Part print with two shaded views. Sizes in mm from the minimum x, y, z corner. A direction names the side the tool comes from. Coordinates: 2 decimals unless noted, no trailing zeros. Order: outer loops, then holes, each group sorted by start corner. A loop starts at its lowest first (then second) coordinate and runs counter-clockwise, first axis right, second up.
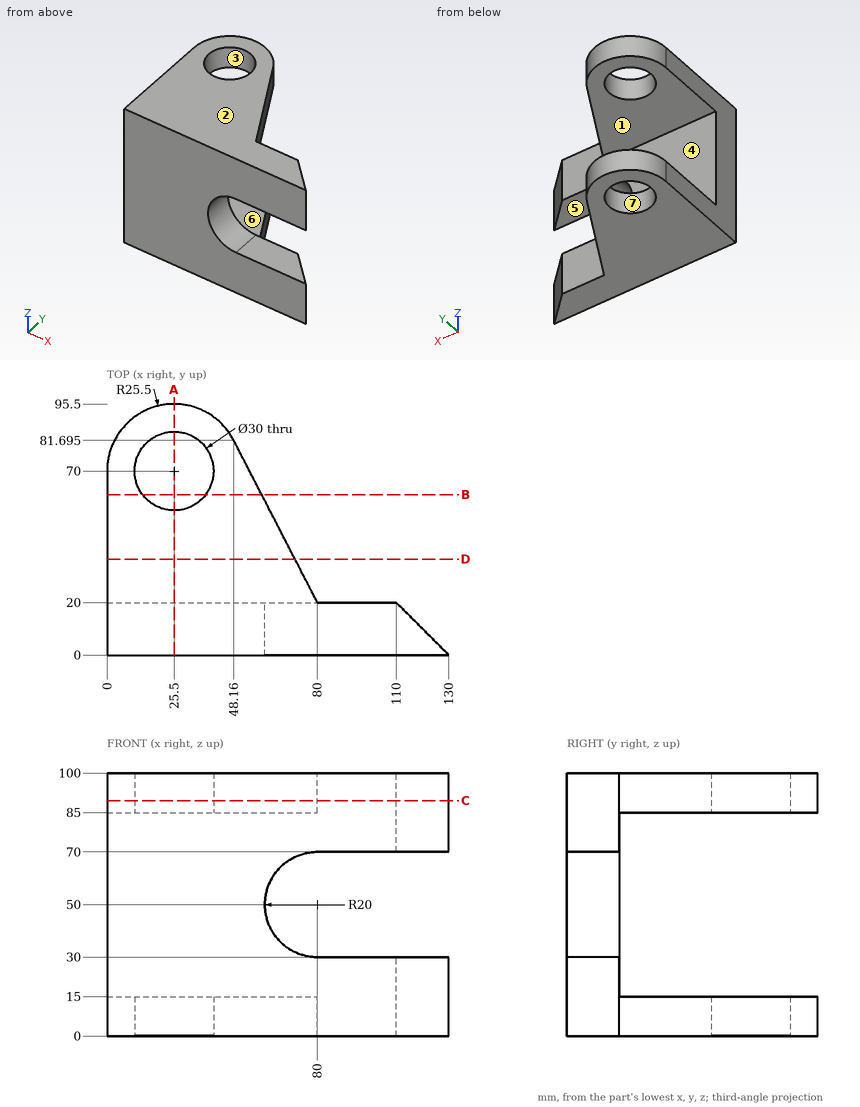
Q1. Wall check: line 1 along Y through (x, z) = (25.5, 9.75); line 2 along Z through (x, y) = (58, 46.5); line 3 along Y through (x, z) = (108, 13). Give the ranges that are in metal, low to high.
Results list:
line 1: y = 0 to 55, 85 to 95.5
line 2: z = 0 to 15, 85 to 100
line 3: y = 0 to 20
Q2. Cut at D-D on y = 36.5. Write the cut outline in (x, z) (1 decimal), and give its area (3 significant figures).
Results list:
outline: (0, 0) - (71.5, 0) - (71.5, 15) - (0, 15) - close; (0, 85) - (71.5, 85) - (71.5, 100) - (0, 100) - close
area: 2,140 mm2
Q3. Pin check, flat tips, straight feed: pin 1 Ø24 at (x, y) = (25.5, 70) entering from +Z; pin 2 Ø8 at (x, z) = (83, 12.5) entering from +Y. Stop position of each tip, or through.
Results list:
pin 1: passes through
pin 2: stops at y = 21.94
Q4. Mould opens along Z. For the marked faces 1, 2, 3 and 4 say: pulls with the +Z half, pulls with the -Z half, needs draft (parallel to the pull), parting line crosses it, or undercut.
Results list:
face 1: undercut
face 2: pulls with the +Z half
face 3: needs draft
face 4: undercut
Q5. Cut at A-A on x = 25.5. Write the cut outline in (y, z).
Results list:
outline: (0, 0) - (55, 0) - (55, 15) - (20, 15) - (20, 85) - (55, 85) - (55, 100) - (0, 100) - close; (85, 0) - (95.5, 0) - (95.5, 15) - (85, 15) - close; (85, 85) - (95.5, 85) - (95.5, 100) - (85, 100) - close
Q6. Which spindle directions (+Z, -Z, +X, -X, +Y, -Y) get a long thin tool onto all of the face, cutting with end or side? Do the marked faces 5, 6 and 7. Say none if no direction does.
Results list:
face 5: +X, +Y, -Y
face 6: +X, -X, +Y
face 7: +Z, -Z
Q7. Cut at B-B on y = 61. Write the cut outline in (x, z).
Results list:
outline: (0, 0) - (13.5, 0) - (13.5, 15) - (0, 15) - close; (0, 85) - (13.5, 85) - (13.5, 100) - (0, 100) - close; (37.5, 0) - (58.84, 0) - (58.84, 15) - (37.5, 15) - close; (37.5, 85) - (58.84, 85) - (58.84, 100) - (37.5, 100) - close
Q8. Cut at C-C on z = 89.5. Write the cut outline in (x, y) (1 decimal), and give its area (3 significant figures).
Results list:
outline: (0, 0) - (130, 0) - (110, 20) - (80, 20) - (48.2, 81.7) arc R25.5 ccw to (0, 70) - close; hole circle Ø30 at (25.5, 70)
area: 6,080 mm2
